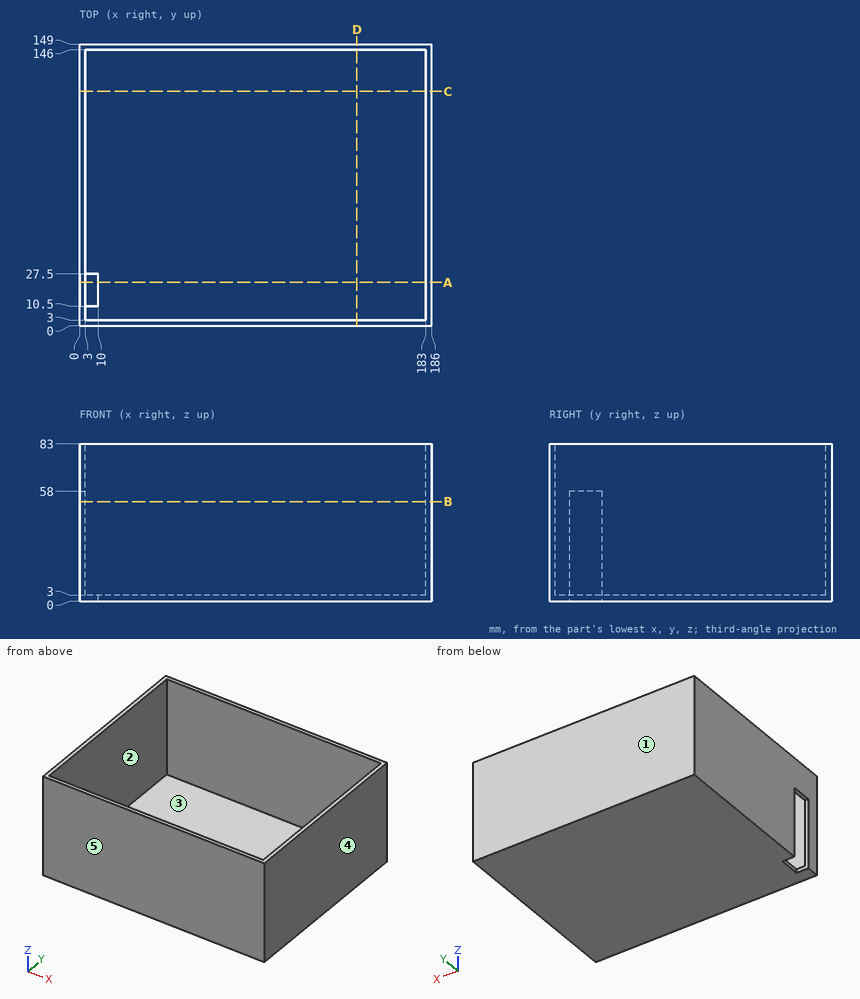
Geometry check sheet. Reference: drawing and pictorial views, mm from the part's lowest x, y, z. A direction names the side the tool comes from. Coordinates: 2 decimals unless noted, no trailing zeros. Write each loop counter-clockwise with the first axis right and the second up, starting at its lowest first coordinate (ties: lowest second). Pieces come first, ordered by that corner, then holes.
Item 1: Access from +Z, -Z, +X, -X, +Y, -Y to the whole of each face (thin tool, end or side, straight path). Record for the marked faces 1 and 2.
Numbers:
face 1: +Z, -Z, +X, -X, +Y
face 2: +Z
Item 2: Depth check by flat-ended pin: pin 1 Ø3.5 at (x, y) = (1, 22.5) entering from -Z; pin 2 Ø3.5 at (y, z) = (20.5, 2) entering from -X; pin 3 Ø5 at (x, y) = (28, 28.5) entering from +Z. Enter the tip coordinate at first touch or a pass-through.
Numbers:
pin 1: stops at z = 58
pin 2: stops at x = 10
pin 3: stops at z = 3
Item 3: Scan lines: probe 1 along Y at (x, z) = (88.5, 47.5); probe 2 along X at (y, z) = (39, 4.5); probe 3 along Z at (x, y) = (154, 59.5). Record each from-to range of solid material in increasing order.
Numbers:
probe 1: y = 0 to 3, 146 to 149
probe 2: x = 0 to 3, 183 to 186
probe 3: z = 0 to 3
Item 4: Cross-section at B-B on z = 52.5. Record the boundary of the cut face in (x, y).
Numbers:
outline: (0, 0) - (186, 0) - (186, 149) - (0, 149) - (0, 27.5) - (3, 27.5) - (3, 146) - (183, 146) - (183, 3) - (3, 3) - (3, 10.5) - (0, 10.5) - close
Item 5: Mould release check, pull along X, two halves, no side actions. Record for the marked faces 3, 4 and 5: released by +X, released by -X, zero draft, split by the parting line, or undercut.
Numbers:
face 3: undercut
face 4: released by +X
face 5: zero draft
Item 6: Cross-section at A-A on y = 23. Record the boundary of the cut face in (x, z).
Numbers:
outline: (0, 58) - (3, 58) - (3, 83) - (0, 83) - close; (10, 0) - (186, 0) - (186, 83) - (183, 83) - (183, 3) - (10, 3) - close
Item 7: Cross-section at D-D on x = 146.5. Record the boundary of the cut face in (y, z).
Numbers:
outline: (0, 0) - (149, 0) - (149, 83) - (146, 83) - (146, 3) - (3, 3) - (3, 83) - (0, 83) - close
Item 8: Cross-section at C-C on y = 124. Record the boundary of the cut face in (x, z), then the cut area to 3 significant figures.
Numbers:
outline: (0, 0) - (186, 0) - (186, 83) - (183, 83) - (183, 3) - (3, 3) - (3, 83) - (0, 83) - close
area: 1,040 mm2
